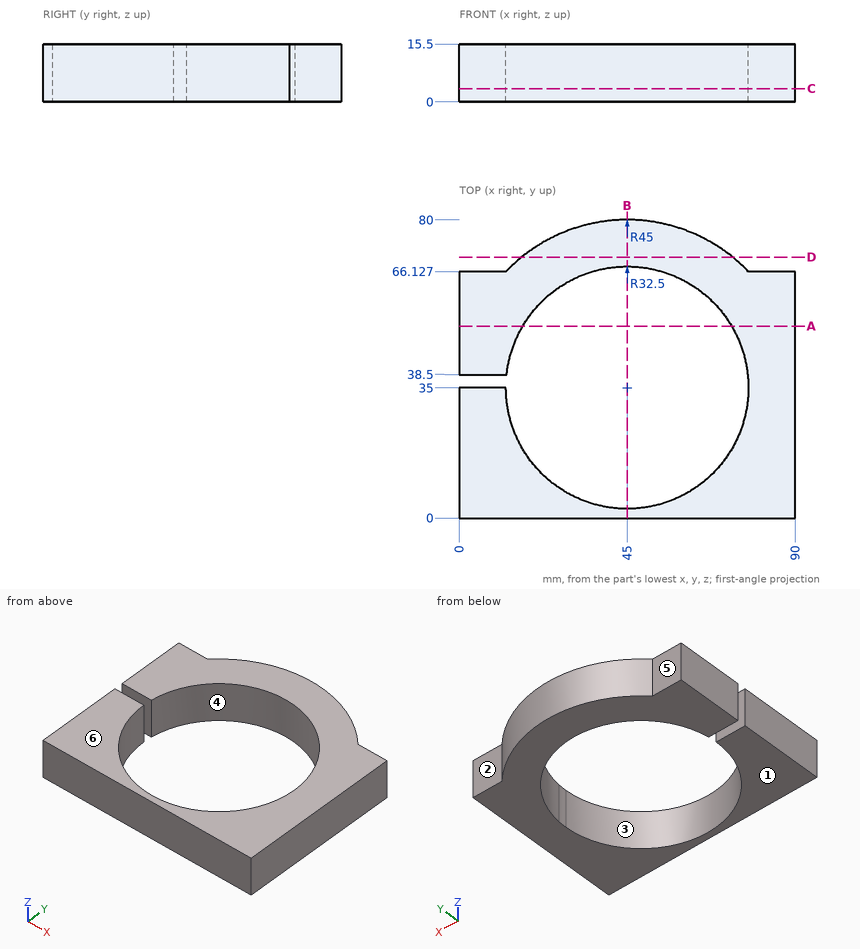
Design review of the part shown in the three views and the two pictorial views. Dimensions are in mm from the part's minimum x, y and z. A direction names the side the tool comes from. Coordinates: 2 decimals unless noted, no trailing zeros. Loops run counter-clockwise (first coordinate to the right, second up) from the corner with the lowest first, then second, coordinate; pieces in that order, holes last. Notation, with made-up numbers: (64, -26) -> (96, -26) arc R20 ccw to (96, -5) -> close; hole circle Ø3 at (10, 40.5). An arc over 180 degrees is marked (long way). Answer as CSV lines item,"result".
Item 1: Take a section at B-B, the plane x = 45. State the section outline as (y, z) points, and give its area (4 significant figures).
Results below:
outline,"(0, 0) -> (2.5, 0) -> (2.5, 15.5) -> (0, 15.5) -> close; (67.5, 0) -> (80, 0) -> (80, 15.5) -> (67.5, 15.5) -> close"
area,"232.5 mm2"
Item 2: Insertion check: pin 1 (2 mm diameter, centred on x = 80.5, z = 4, fed in from +Y); pin 2 (4 mm diameter, centred on y = 72, z = 11, fed in from +X) (1 decimal); pin 3 (8 mm diameter, centred on y = 24.5, z = 13, fed in from -X). Each pin has a flat end and moves straight along its axis. Give the tip position at first contact, or say it passes through.
Results below:
pin 1,"stops at y = 66.13"
pin 2,"stops at x = 73.3"
pin 3,"stops at x = 0"
Item 3: Draft analysis for pull direction Y (two halves, no side actions). For the marked faces 1, 2, 3 and 4, state which applies: +Y half, -Y half, draft (parallel to the pull), parting line (faces both ways), or undercut.
Results below:
face 1,"draft"
face 2,"+Y half"
face 3,"undercut"
face 4,"undercut"
Item 4: Take a section at A-A, the plane y = 51.5. State the section outline as (x, z) points.
Results below:
outline,"(0, 0) -> (17, 0) -> (17, 15.5) -> (0, 15.5) -> close; (73, 0) -> (90, 0) -> (90, 15.5) -> (73, 15.5) -> close"
Item 5: For L1, parallel to Y at x = 5.5, z = 8.5; L2, parallel to Y at x = 81.5, z = 12.5; L3, parallel to X at y = 42.5, z = 11, list the stretches that pass through material, from the lowest coordinate up.
Results below:
L1,"y = 0 to 35, 38.5 to 66.13"
L2,"y = 0 to 66.13"
L3,"x = 0 to 13.38, 76.62 to 90"
Item 6: Machinability: for the marked faces 5 and 6, which of the approach directions +Z, -Z, +X, -X, +Y, -Y give a long, thin tool a straight path to every point of the face, cutting with its end or side? Answer none if there is none.
Results below:
face 5,"+Z, -Z, -X, +Y"
face 6,"+Z, +X, -X, +Y, -Y"
Item 7: Take a section at C-C, the plane z = 3.5. State the section outline as (x, y) points.
Results below:
outline,"(0, 0) -> (90, 0) -> (90, 66.13) -> (77.5, 66.13) arc R45 ccw to (12.5, 66.13) -> (0, 66.13) -> (0, 38.5) -> (12.69, 38.5) arc R32.5 cw to (77.31, 38.5) arc R32.5 cw to (77.5, 35) arc R32.5 cw to (12.5, 35) -> (0, 35) -> close"
Item 8: Take a section at D-D, the plane y = 70. State the section outline as (x, z) points, and give its area (3 significant figures).
Results below:
outline,"(16.72, 0) -> (73.28, 0) -> (73.28, 15.5) -> (16.72, 15.5) -> close"
area,"877 mm2"
